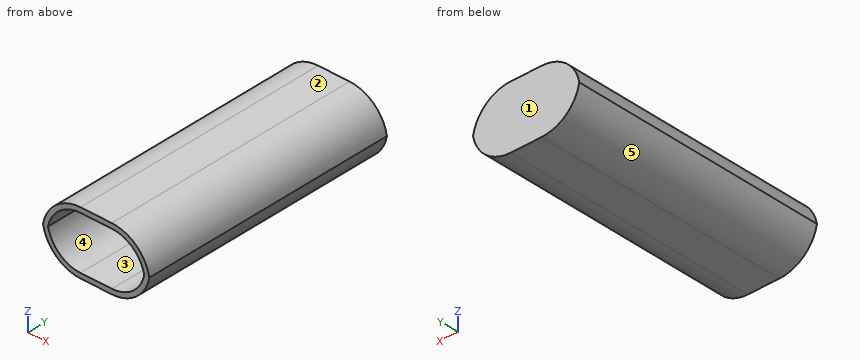
from build123d import *

# Parameters (mm, degrees)
F0_W        = 55.4167628288
F0_H        = 32.3319099844
F1_DEPTH    = 133.096
F2_T1_DEPTH = 231.2096391748
F3_T        = -2.54


# Not quite as in the source:
# - a fillet or chamfer that OpenCascade refuses, or shapes differently, is made with other operations: its cross-section is extruded or revolved along the edge and cut away or added


with BuildPart() as f1:
    # F0 (on Front) → F1 (new body)
    with BuildSketch(Plane.XZ):
        with Locations((-27.7083814144, 16.1659549922)):
            Rectangle(F0_W, F0_H)
    extrude(amount=F1_DEPTH)

    # F2: fillet of radius 19.622727835 on 4 edges, made by hand

    # F2_s2 → F2_t1 (cut)
    with BuildSketch(Plane.XZ.offset(-49.0568195874)):
        with BuildLine():
            ThreePointArc((-35.7940349939, 32.3319099844), (-49.6693989113, 26.5845460669), (-55.4167628288, 12.7091821494))
            Line((-55.4167628288, 12.7091821494), (-55.4167628288, 32.3319099844))
            Line((-55.4167628288, 32.3319099844), (-35.7940349939, 32.3319099844))
        make_face()
        with BuildLine():
            ThreePointArc((0, 12.7091821494), (-5.7473639175, 26.5845460669), (-19.622727835, 32.3319099844))
            Line((-19.622727835, 32.3319099844), (0, 32.3319099844))
            Line((0, 32.3319099844), (0, 12.7091821494))
        make_face()
        with BuildLine():
            ThreePointArc((-19.622727835, 0), (-5.7473639175, 5.7473639175), (0, 19.622727835))
            Line((0, 19.622727835), (0, 0))
            Line((0, 0), (-19.622727835, 0))
        make_face()
        with BuildLine():
            ThreePointArc((-35.7940349939, 0), (-49.6693989113, 5.7473639175), (-55.4167628288, 19.622727835))
            Line((-55.4167628288, 19.622727835), (-55.4167628288, 0))
            Line((-55.4167628288, 0), (-35.7940349939, 0))
        make_face()
    extrude(amount=F2_T1_DEPTH, mode=Mode.SUBTRACT)

    # F3
    f3_openings = [f1.faces().sort_by_distance(p)[0] for p in [
        (-27.708381, -133.096, 16.165955),
    ]]
    offset(amount=F3_T, openings=f3_openings)


solid = f1.part
Geometry: final body of the model. Coordinates: model frame, mm. Face numbers are marked on the shaded views. A direction names the side the tool comes from. Give positions to 0.01 mm unless a question says otherwise; leave off trailing zeros. Write each loop counter-clockwise with the first axis right and the second up, starting at its lowest first coordinate (ties: lowest second). Pieces come first, ordered by that corner, then holes.
(1) Cut plane C-C, the plane z = 12.5. Return loops of the section in (x, y), then the cut area to 3 significant figures.
(2) Mould query, pull axis Z, two halves, no side actions, for the marked faces 1, 2 and 3. Classes: released by +Z, released by -Z, zero draft, split by the parting line, or undercut.
(3) Cut plane B-B, the plane x = -23.5. Return loops of the section in (y, z).
(4) Cut plane A-A, the plane y = -20. Return loops of the section in (x, z), then the cut area to 3 significant figures.
(5) Access query for the marked faces 4 and 5. Directions: +Z, -Z, +X, -X, +Y, -Y. A direction counts if a zero-diameter tool reaches every point of the face in a straight line with its end or side. Return the directions, or none.
(6) Ray query, line 1 (Z direction, x = -19, y = -115); line 2 (Z direction, x = -30.5, y = -111); line 3 (X direction, y = -70.5, z = 6.5). Return the intervals inside material, ascending.
(7) First-contact query: P1, Ø10, axis at y = -117, z = 9, coming from the -X side; P2, Ø8, axis at x = -19.5, z = 18, coming from the -Y side; P3, Ø8, axis at y = -80.5, z = 8, coming from the +X side. Flat tips, straight axial feed; report the tip coordinate or a pass-through.
Values follow:
1. outline: (-54.08, -133.1) - (-51.32, -133.1) - (-51.32, -2.54) - (-4.1, -2.54) - (-4.1, -133.1) - (-1.34, -133.1) - (-1.34, 0) - (-54.08, 0) - close
1. area: 854 mm2
2. face 1: zero draft
2. face 2: released by +Z
2. face 3: undercut
3. outline: (-133.1, 0) - (0, 0) - (0, 32.33) - (-133.1, 32.33) - (-133.1, 29.79) - (-2.54, 29.79) - (-2.54, 2.54) - (-133.1, 2.54) - close
4. outline: (-55.11, 16.17) arc R19.62 ccw to (-35.79, 0) - (-19.62, 0) arc R19.62 ccw to (-0.31, 16.17) arc R19.62 ccw to (-19.62, 32.33) - (-35.79, 32.33) arc R19.62 ccw to start; hole (-52.52, 16.17) arc R17.08 ccw to (-35.79, 2.54) - (-19.62, 2.54) arc R17.08 ccw to (-2.89, 16.17) arc R17.08 ccw to (-19.62, 29.79) - (-35.79, 29.79) arc R17.08 ccw to start
4. area: 340 mm2
5. face 4: -Y
5. face 5: -Z, -X, +Y, -Y
6. line 1: z = 0.01 to 2.55, 29.78 to 32.32
6. line 2: z = 0 to 2.54, 29.79 to 32.33
6. line 3: x = -50.38 to -46.73, -8.69 to -5.03
7. P1: stops at x = -54.59
7. P2: stops at y = -2.54
7. P3: stops at x = -1.54
